from build123d import *

# Parameters (mm, degrees)
SKETCH1_W           = 95
SKETCH1_H           = 35
BOSS_EXTRUDE1_DEPTH = 3
CUT_EXTRUDE1_REACH  = 52.71
SKETCH3_R           = 8
CUT_EXTRUDE2_REACH  = 52.71
SKETCH4_R           = 1.5
SKETCH5_W           = 95
SKETCH5_H           = 4
BOSS_EXTRUDE2_DEPTH = 3
CUT_EXTRUDE3_REACH  = 54.225
SKETCH6_W           = 10
SKETCH6_H           = 4.2
CUT_EXTRUDE4_REACH  = 54.225
SKETCH7_R           = 1.5
CUT_EXTRUDE5_REACH  = 54.225
SKETCH8_W           = 105.539235452
SKETCH8_H           = 51.644684014
SKETCH8_W_2         = 83
SKETCH8_H_2         = 32
FILLET1_R           = 5


with BuildPart() as part:
    # Sketch1 → Boss-Extrude1 (new body)
    with BuildSketch(Plane(origin=(0, 0, 0), x_dir=(1, 0, 0), z_dir=(0, 1, 0))):
        Rectangle(SKETCH1_W, SKETCH1_H)
    extrude(amount=BOSS_EXTRUDE1_DEPTH)

    # Sketch3 → Cut-Extrude1 (cut, up to next)
    with BuildSketch(Plane.XZ, mode=Mode.PRIVATE) as cut_extrude1_sk1:
        with Locations(Location((-13, 1.5, 0), (0, 0, 270))):
            Circle(SKETCH3_R)
    cut_extrude1_tool1 = extrude(cut_extrude1_sk1.sketch, amount=-CUT_EXTRUDE1_REACH, mode=Mode.PRIVATE) & part.part
    # Sketch3 → Cut-Extrude1 (cut, up to next)
    with BuildSketch(Plane.XZ, mode=Mode.PRIVATE) as cut_extrude1_sk2:
        with Locations(Location((13, 1.5, 0), (0, 0, 270))):
            Circle(SKETCH3_R)
    cut_extrude1_tool2 = extrude(cut_extrude1_sk2.sketch, amount=-CUT_EXTRUDE1_REACH, mode=Mode.PRIVATE) & part.part
    add(cut_extrude1_tool1.solids().sort_by_distance((-13, 0, 1.5))[0], mode=Mode.SUBTRACT)
    add(cut_extrude1_tool2.solids().sort_by_distance((13, 0, 1.5))[0], mode=Mode.SUBTRACT)

    # Sketch4 → Cut-Extrude2 (cut, up to next)
    with BuildSketch(Plane(origin=(0, 0, 0), x_dir=(1, 0, 0), z_dir=(0, 1, 0)), mode=Mode.PRIVATE) as cut_extrude2_sk1:
        with Locations(Location((-37.75, -12.5, 0), (0, 0, 90))):
            Circle(SKETCH4_R)
    cut_extrude2_tool1 = extrude(cut_extrude2_sk1.sketch, amount=CUT_EXTRUDE2_REACH, mode=Mode.PRIVATE) & part.part
    # Sketch4 → Cut-Extrude2 (cut, up to next)
    with BuildSketch(Plane(origin=(0, 0, 0), x_dir=(1, 0, 0), z_dir=(0, 1, 0)), mode=Mode.PRIVATE) as cut_extrude2_sk2:
        with Locations(Location((27.75, -12.5, 0), (0, 0, 90))):
            Circle(SKETCH4_R)
    cut_extrude2_tool2 = extrude(cut_extrude2_sk2.sketch, amount=CUT_EXTRUDE2_REACH, mode=Mode.PRIVATE) & part.part
    # Sketch4 → Cut-Extrude2 (cut, up to next)
    with BuildSketch(Plane(origin=(0, 0, 0), x_dir=(1, 0, 0), z_dir=(0, 1, 0)), mode=Mode.PRIVATE) as cut_extrude2_sk3:
        with Locations(Location((22.75, 12.5, 0), (0, 0, 90))):
            Circle(SKETCH4_R)
    cut_extrude2_tool3 = extrude(cut_extrude2_sk3.sketch, amount=CUT_EXTRUDE2_REACH, mode=Mode.PRIVATE) & part.part
    # Sketch4 → Cut-Extrude2 (cut, up to next)
    with BuildSketch(Plane(origin=(0, 0, 0), x_dir=(1, 0, 0), z_dir=(0, 1, 0)), mode=Mode.PRIVATE) as cut_extrude2_sk4:
        with Locations(Location((-32.75, 12.5, 0), (0, 0, 90))):
            Circle(SKETCH4_R)
    cut_extrude2_tool4 = extrude(cut_extrude2_sk4.sketch, amount=CUT_EXTRUDE2_REACH, mode=Mode.PRIVATE) & part.part
    add(cut_extrude2_tool1.solids().sort_by_distance((-37.75, 0, 12.5))[0], mode=Mode.SUBTRACT)
    add(cut_extrude2_tool2.solids().sort_by_distance((27.75, 0, 12.5))[0], mode=Mode.SUBTRACT)
    add(cut_extrude2_tool3.solids().sort_by_distance((22.75, 0, -12.5))[0], mode=Mode.SUBTRACT)
    add(cut_extrude2_tool4.solids().sort_by_distance((-32.75, 0, -12.5))[0], mode=Mode.SUBTRACT)

    # Sketch5 → Boss-Extrude2 (add)
    with BuildSketch(Plane(origin=(0, 0, 0), x_dir=(1, 0, 0), z_dir=(0, 1, 0))):
        with Locations((0, -19.5)):
            Rectangle(SKETCH5_W, SKETCH5_H)
        with Locations((0, 19.5)):
            Rectangle(SKETCH5_W, SKETCH5_H)
    extrude(amount=BOSS_EXTRUDE2_DEPTH)

    # Sketch6 → Cut-Extrude3 (cut, up to next)
    with BuildSketch(Plane(origin=(0, 0, 0), x_dir=(1, 0, 0), z_dir=(0, 1, 0)), mode=Mode.PRIVATE) as cut_extrude3_sk1:
        with Locations((-30.75, 4.9)):
            Rectangle(SKETCH6_W, SKETCH6_H)
    cut_extrude3_tool1 = extrude(cut_extrude3_sk1.sketch, amount=CUT_EXTRUDE3_REACH, mode=Mode.PRIVATE) & part.part
    # Sketch6 → Cut-Extrude3 (cut, up to next)
    with BuildSketch(Plane(origin=(0, 0, 0), x_dir=(1, 0, 0), z_dir=(0, 1, 0)), mode=Mode.PRIVATE) as cut_extrude3_sk2:
        with Locations((30.75, 4.9)):
            Rectangle(SKETCH6_W, SKETCH6_H)
    cut_extrude3_tool2 = extrude(cut_extrude3_sk2.sketch, amount=CUT_EXTRUDE3_REACH, mode=Mode.PRIVATE) & part.part
    add(cut_extrude3_tool1.solids().sort_by_distance((-30.75, 0, -4.9))[0], mode=Mode.SUBTRACT)
    add(cut_extrude3_tool2.solids().sort_by_distance((30.75, 0, -4.9))[0], mode=Mode.SUBTRACT)

    # Sketch7 → Cut-Extrude4 (cut, up to next)
    with BuildSketch(Plane.XZ, mode=Mode.PRIVATE) as cut_extrude4_sk1:
        with Locations((-5, 2.201101087)):
            Circle(SKETCH7_R)
    cut_extrude4_tool1 = extrude(cut_extrude4_sk1.sketch, amount=-CUT_EXTRUDE4_REACH, mode=Mode.PRIVATE) & part.part
    # Sketch7 → Cut-Extrude4 (cut, up to next)
    with BuildSketch(Plane.XZ, mode=Mode.PRIVATE) as cut_extrude4_sk2:
        with Locations((5, 2.201101087)):
            Circle(SKETCH7_R)
    cut_extrude4_tool2 = extrude(cut_extrude4_sk2.sketch, amount=-CUT_EXTRUDE4_REACH, mode=Mode.PRIVATE) & part.part
    add(cut_extrude4_tool1.solids().sort_by_distance((-5, 0, 2.201101))[0], mode=Mode.SUBTRACT)
    add(cut_extrude4_tool2.solids().sort_by_distance((5, 0, 2.201101))[0], mode=Mode.SUBTRACT)

    # Sketch8 → Cut-Extrude5 (cut, up to next)
    with BuildSketch(Plane(origin=(0, 0, 0), x_dir=(1, 0, 0), z_dir=(0, 1, 0)), mode=Mode.PRIVATE) as cut_extrude5_sk1:
        Rectangle(SKETCH8_W, SKETCH8_H)
        Rectangle(SKETCH8_W_2, SKETCH8_H_2, mode=Mode.SUBTRACT)
    cut_extrude5_tool1 = extrude(cut_extrude5_sk1.sketch, amount=CUT_EXTRUDE5_REACH, mode=Mode.PRIVATE) & part.part
    add(cut_extrude5_tool1.solids().sort_by_distance((0, 0, -24.647365))[0], mode=Mode.SUBTRACT)

    # Fillet1
    fillet1_edges = [part.edges().sort_by_distance(p)[0] for p in [
        (41.5, 1.5, -16),
        (-41.5, 1.5, -16),
        (-41.5, 1.5, 16),
        (41.5, 1.5, 16),
    ]]
    fillet(fillet1_edges, radius=FILLET1_R)


solid = part.part
The listing builds one solid part. Answer for the finished solid, in the listing's coordinates (mm). A direction names the side the tool comes from. Give positions to 0.01 mm unless a question says otherwise; leave off trailing zeros. Order: outer loops, then holes, each group sorted by start corner. A loop starts at its lowest first (then second) coordinate and runs counter-clockwise, first axis right, second up. Notation, with made-up numbers: (-1, -34) - (11, -34) arc R13 cw to (11, -28) - close; hole circle Ø10 at (76.25, -12). An arc over 180 degrees is marked (long way). One line per item, written item: value. Start each with the question number.
1) A tool of negligible diameter and unlimited length cuts with its end or side. For faces 1 (the face through (-3.503, 1.479, 2.297)), 2 (the face through (40, 1.52, -14.57)), from which of +Z, -Z, +X, -X, +Y, -Y can it reach the whole face along a straight path? Write none if from no direction.
2) Find the intervals of material crossed by L1, parallel to Z at x = 5, y = 0.8; L2, parallel to X at y = 2.5, z = -5; L3, parallel to X at y = 2.4, z = 8.5, in increasing order.
3) A cutting plane is placed at A-A on x = 22.75. Give the vertices of the cut face in (y, z), then the cut area to 3 significant figures.
4) A cutting plane is placed at D-D on y = 2.25. State how many separate pieces and enclosed holes the cut face has, then the cut area to 3 significant figures.
5) A cutting plane is placed at C-C on x = -32.75. Give the vertices of the cut face in (y, z).
6) The mould has two halves that part along X. Classify faces 3 (the face through (-41.5, 1, 0)), 4 (the face through (31, 1, -2.8)), 5 (the face through (-1, 3, 0)): released by +X, released by -X, zero draft, split by the parting line, or undercut.
7) A cutting plane is placed at B-B on z = 12. Give the vertices of the cut face in (x, y), then the cut area to 3 significant figures.
8) Given pin 1 Ø1.8 at (x, z) = (-5, 2.2) entering from -Y, flat-ended and moving along its own axis, determine where the tip first touches the part or whether it passes through.
Answer sheet:
1. face 1: +Y, -Y
1. face 2: -Z, +X, +Y, -Y
2. L1: z = -16 to 0.7, 3.7 to 16
2. L2: x = -41.5 to -35.75, -25.75 to -17.66, -8.34 to 8.34, 17.66 to 25.75, 35.75 to 41.5
2. L3: x = -41.5 to -16.87, -9.13 to 9.13, 16.87 to 41.5
3. outline: (0, -16) - (3, -16) - (3, -14) - (0, -14) - close; (0, -11) - (3, -11) - (3, 16) - (0, 16) - close
3. area: 87.0 mm2
4. separate pieces: 1
4. enclosed holes: 8
4. area: 2,110 mm2
5. outline: (0, -16) - (3, -16) - (3, -14) - (0, -14) - close; (0, -11) - (3, -11) - (3, -7) - (0, -7) - close; (0, -2.8) - (3, -2.8) - (3, 16) - (0, 16) - close
6. face 3: released by -X
6. face 4: undercut
6. face 5: zero draft
7. outline: (-41.4, 0) - (-39.16, 0) - (-39.16, 3) - (-41.4, 3) - close; (-36.34, 0) - (26.34, 0) - (26.34, 3) - (-36.34, 3) - close; (29.16, 0) - (41.4, 0) - (41.4, 3) - (29.16, 3) - close
7. area: 231 mm2
8. pin 1: passes through
